Autodesk Inventor part; units mm, degrees
ref_plane "Work Plane1" through (0, 13, 0) normal (0, -1, 0) x (1, 0, 0)
ref_plane "Work Plane2" through (-11, 0, -10.875) normal (1, 0, 0) x (0, 0, -1)
ref_plane "YZ Plane" through (0, 0, 0) normal (1, 0, 0) x (0, 1, 0)
sketch "Sketch1" plane through (0, 0, 0) normal (0, 1, 0) x (-1, 0, 0)
  arc A0 (0, -10.875) -> (0, 10.875) centre (0, 0) ccw
  line L0 (0, -10.875) -> (0, 10.875)
  dimension "d0" = 21.75
extrude "Extrusion1" add sketch "Sketch1" along normal blind 20
sketch "Sketch2" plane through (0, 20, 0) normal (0, 1, 0) x (1, 0, 0)
  circle A0 centre (0, 0) radius 2
  dimension "d3" = 4
extrude "Extrusion2" cut sketch "Sketch2" against normal through all
ref_plane "Work Plane1" through (0, 13, 0) normal (0, -1, 0) x (1, 0, 0)
sketch "Sketch3" plane through (0, 13, 0) normal (0, -1, 0) x (1, 0, 0)
  line L0 (-2, -7.5208) -> (2, -7.5208) construction
  line L1 (2, -7.5208) -> (2, 8.0151) construction
  line L2 (2, 8.0151) -> (-2, 8.0151) construction
  line L3 (-2, 8.0151) -> (-2, -7.5208) construction
  line L4 (2.6754, -7.3078) -> (5.9521, -5.0135) construction
  line L5 (5.9521, -5.0135) -> (-2.959, 7.7128) construction
  line L6 (-2.959, 7.7128) -> (-6.2356, 5.4185) construction
  line L7 (-6.2356, 5.4185) -> (2.6754, -7.3078) construction
  line L8 (5.9521, 5.0135) -> (2.6754, 7.3078) construction
  line L9 (2.6754, 7.3078) -> (-6.2356, -5.4185) construction
  line L10 (-6.2356, -5.4185) -> (-2.959, -7.7128) construction
  line L11 (-2.959, -7.7128) -> (5.9521, 5.0135) construction
  line L12 (-5.1857, 3.919) -> (-2.4415, 0)
  line L13 (-5.1857, -3.919) -> (-2.4415, 0)
  line L14 (0, 10.875) -> (0, 2)
  line L15 (0, 6.4375) -> (0, -6.5)
  arc A0 (1.9091, -6.2133) -> (2, -6.1847) centre (0, 0) ccw
  arc A1 (2, 6.1847) -> (1.9091, 6.2133) centre (0, 0) ccw
  arc A2 (0, 6.5) -> (-5.1857, 3.919) centre (0, 0) ccw
  arc A3 (-5.1857, -3.919) -> (0, -6.5) centre (0, 0) ccw
  point P0 (2, 7.5208)
  point P1 (-2, -8.0151)
  dimension "d29" = 4
  dimension "d32" = 35
  dimension "d36" = 145
extrude "Extrusion3" cut sketch "Sketch3" along normal blind 4.1
sketch "Sketch4" plane through (0, 20, 0) normal (0, 1, 0) x (1, 0, 0)
  line L0 (0, 0) -> (-10.2573, 10.2573) construction
  line L1 (0, 0) -> (14.5061, 0) construction
  point P0 (-5.1265, 5.1265)
  dimension "d38" = 7.25
  dimension "d39" = 225
hole "Hole1" at (-5.1265, 20, -5.1265) direction (0, -1, 0) diameter 1.567 depth 5 tip angle 118
sketch "Sketch5" plane through (0, 0, 10.875) normal (1, 0, 0) x (0, 0, -1)
  line L0 (8.875, 8.9) -> (4.375, 8.9)
  line L1 (8.875, 0) -> (8.875, 8.9)
  point P0 (10.875, 0)
  point P1 (5.375, 4.4)
  dimension "d47" = 4.5
  dimension "d50" = 3.5
hole "Hole2" at (0, 4.4, 5.5) direction (-1, 0, 0) diameter 2.459 depth 5 tip angle 118
sketch "Sketch6" plane through (0, 0, -10.875) normal (1, 0, 0) x (0, 0, -1)
  line L0 (-8.875, 8.9) -> (-8.875, 0)
  line L1 (-4.375, 8.9) -> (-8.875, 8.9)
  point P0 (-10.875, 0)
  point P1 (-5.375, 4.4)
  dimension "d58" = 3.5
  dimension "d59" = 4.5
hole "Hole3" at (0, 4.4, -5.5) direction (-1, 0, 0) diameter 3 end through all
ref_plane "Work Plane2" through (-11, 0, -10.875) normal (1, 0, 0) x (0, 0, -1)
sketch "Sketch7" plane through (-11, 0, -10.875) normal (1, 0, 0) x (0, 0, -1)
  circle A0 centre (-5.375, 4.4) radius 1.5
  point P0 (-10.875, 0)
hole "Hole4" at (-11, 4.4, -5.5) direction (1, 0, 0) diameter 3 end through all counterbore diameter 4 counterbore depth 6
sketch "Sketch8" plane through (0, 0, 0) normal (0, -1, 0) x (1, 0, 0)
  circle A0 centre (0, 0) radius 2.7 construction
  line L0 (0, 3) -> (0, 2.4) construction
  line L1 (0, 6.5) -> (0, 2)
  arc A1 (-3, 1.6) -> (-3, -1.6) centre (0, 0) ccw
  arc A2 (-2.4, -2.4083) -> (-1.6, 3) centre (0, 0) ccw
  line L2 (-2.4, 9) -> (-3, 9)
  line L3 (-3, 9) -> (-3, 1.6)
  arc A3 (-3, 1.6) -> (-2.4, 2.4083) centre (0, 0) ccw
  arc A4 (-2.4, -2.4083) -> (-2.4, 2.4083) centre (0, 0) ccw
  arc A5 (-3, 1.6) -> (-3, -1.6) centre (0, 0) ccw
  line L4 (-2.4, 2.4083) -> (-2.4, 9)
  point P0 (0, 2.7)
  dimension "d76" = 5.4
  dimension "d80" = 0
  dimension "d88" = 0.6
  dimension "d89" = 9
extrude "Extrusion4" cut sketch "Sketch8" against normal blind 1
sketch "Sketch9" plane through (0, 8.9, 0) normal (0, 1, 0) x (1, 0, 0)
  circle A0 centre (0, 0) radius 2.5
  dimension "d90" = 5
extrude "Extrusion5" cut sketch "Sketch9" against normal blind 5 and the other way blind 8
sketch "Sketch10" plane through (0, 0, 0) normal (0, 0, 1) x (1, 0, 0)
  line L0 (-10.875, 0) -> (-10.875, 20)
  line L1 (-10.875, 12.5) -> (-7.875, 12.5)
  line L2 (-7.875, 12.5) -> (-7.875, 7.5)
  line L3 (-7.875, 7.5) -> (-10.875, 7.5)
  line L4 (-10.875, 7.5) -> (-10.875, 12.5)
  line L5 (0, 20) -> (-10.875, 20)
  point P0 (0, 0)
  dimension "d95" = 3
  dimension "d96" = 7.5
  dimension "d97" = 5
extrude "Extrusion6" cut sketch "Sketch10" along normal through all both and the other way through all
properties part number "HalfEncoderSupprt"
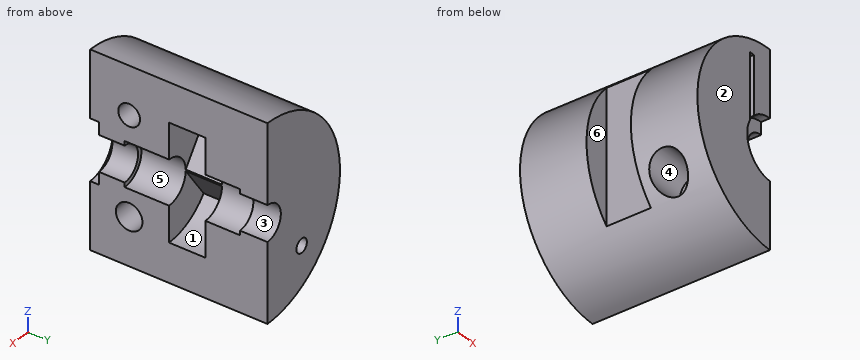
Verification items for the finished model (mm, model axes). Face numbers are marked on the shaded views. A direction names the side the tool comes from. Coordinates: 2 decimals unless noted, no trailing zeros. Order: outer loops, then holes, each group sorted by start corner. A loop starts at its lowest first (then second) coordinate and runs counter-clockwise, first axis right, second up. Notation, with made-up numbers: (45.25, -14.75) -> (49.25, -14.75) arc R4 cw to (49.25, -7.75) -> close; hole circle Ø9 at (8, 56). An arc over 180 degrees is marked (long way). Answer as CSV lines item,"result". Start each with the question number.
1) Gauge pin test, flat ends, axial feed: pin 1 Ø2.5 at (y, z) = (4.4, -5.5) entering from -X; pin 2 Ø3 at (x, z) = (-4.5, -5.5) entering from -Y; pin 3 Ø0.8 at (y, z) = (0.5, 7) entering from -X; pin 4 Ø1 at (x, y) = (-7, 10) entering from +Z. Record the tip position at first contact, or that the pin passes through.
2) Material ranges on L1, parallel to Y at x = -2.25, z = 5.5; L2, parallel to Y at x = -2.95, z = 5.5; L3, parallel to Z at x = -3, y = 4.4, recorded low to high. Write a range as [from, to].
3) Set-up check for the marked faces 4, 5 and 6: record each of +Z, -Z, +X, -X, +Y, -Y from which the full face is reachable in a straight line by a thin tool's end or side.
4) Cross-section at D-D, the plane y = 10.25. Record the boundary of the cut face in (x, z) (3 decimals), then the cut area to 3 significant figures.
5) Cross-section at A-A, the plane x = -9. Record the boundary of the cut face in (y, z), then the cut area to 3 significant figures.
6) Cross-section at C-C, the plane z = -1.25. Record the boundary of the cut face in (x, y) (3 decimals).
7) Release check for a two-part mould opening along Y. For the marked faces 1, 2 and 3 record: released by +Y, released by -Y, zero draft, split by the parting line, or undercut.
Conclusion:
1,pin 1,"passes through"
1,pin 2,"stops at y = 0"
1,pin 3,"stops at x = -8.64"
1,pin 4,"stops at z = 8.72"
2,L1,"y = [0, 3.17], [5.63, 8.9], [13, 20]"
2,L2,"y = [1, 3.17], [5.63, 8.9], [13, 20]"
2,L3,"z = [-10.45, -7], [-4, 4.27], [6.73, 10.45]"
3,face 4,"-X"
3,face 5,"+X"
3,face 6,"+Z, -Z, -X"
4,outline,"(-7.875, -7.5) arc R10.875 ccw to (0, -10.875) -> (0, -6.5) arc R6.5 cw to (-5.186, -3.919) -> (-2.499, -0.082) arc R2.5 cw to (-2.499, 0.082) -> (-5.186, 3.919) arc R6.5 cw to (0, 6.5) -> (0, 10.875) arc R10.875 ccw to (-7.875, 7.5) -> close"
4,area,"106 mm²"
5,outline,"(0, -6.1) -> (2.49, -6.1) arc R2 cw (long way) to (6.31, -6.1) -> (7.5, -6.1) -> (7.5, 6.1) -> (0, 6.1) -> close; (12.5, -6.1) -> (20, -6.1) -> (20, 6.1) -> (12.5, 6.1) -> close"
5,area,"174 mm²"
6,outline,"(-10.803, 0) -> (-3.162, 0) -> (-3.162, 1) -> (-1.561, 1) -> (-1.561, 3.9) -> (-2.165, 3.9) -> (-2.165, 8.9) -> (-3.317, 8.9) -> (-3.317, 13) -> (-2.165, 13) -> (-2.165, 16.9) -> (-1.561, 16.9) -> (-1.561, 20) -> (-10.803, 20) -> (-10.803, 12.5) -> (-7.875, 12.5) -> (-7.875, 7.5) -> (-10.803, 7.5) -> close"
7,face 1,"undercut"
7,face 2,"released by -Y"
7,face 3,"zero draft"
